Verification items for the finished model (mm, model axes). Round coordinates to 2 decimals unless told otherwise and drop trailing zeros. Write each loop counter-clockwise with the first axis right and the second up, starting at its lowest first coordinate (ties: lowest second). Pieces come first, ordered by that corner, then holes. Notation, with made-up numbers: (48.5, 29) -> (63.5, 29) arc R21 cw to (63.5, 49) -> close; hole circle Ø10 at (3.25, 45). An arc over 180 degrees is marked (long way). Answer as a JSON object with one key per item and string values. Group by question number.
(1) Sectioned sample at A-A on x = 22. Record the cut outline in (y, z), and give its area (3 significant figures).
(2) Sectioned sample at B-B on z = 3.2. Record the cut outline in (x, y), and give its area (3 significant figures).
(3) Sectioned sample at C-C on y = -11.5. Record the cut outline in (x, z).
(4) Scan lines: L1, parallel to Y at x = 17, z = 1.8; L2, parallel to X at y = -11.5, z = 4.5; L3, parallel to X at y = 10.5, z = 2.65. Record each from-to range of solid material in increasing order. Write a range as from..to.
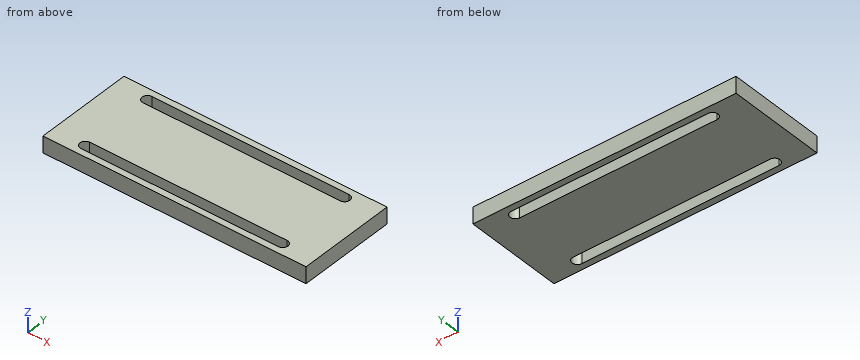
Autodesk Inventor part; units mm, degrees
ref_plane "YZ Plane" through (0, 0, 0) normal (1, 0, 0) x (0, 1, 0)
ref_plane "XZ Plane" through (0, 0, 0) normal (0, 1, 0) x (-1, 0, 0)
ref_plane "XY Plane" through (0, 0, 0) normal (0, 0, 1) x (1, 0, 0)
sketch "スケッチ1" plane through (0, 0, 0) normal (0, 0, 1) x (1, 0, 0)
  line L0 (-40, 15) -> (40, 15)
  line L1 (40, 15) -> (40, -15)
  line L2 (40, -15) -> (-40, -15)
  line L3 (-40, -15) -> (-40, 15)
  point P0 (0, 0)
  dimension "d0" = 80
  dimension "d1" = 40
  dimension "d2" = 30
  dimension "d3" = 15
extrude "押し出し1" add sketch "スケッチ1" along normal blind 5
sketch "スケッチ2" plane through (0, 0, 5) normal (0, 0, 1) x (1, 0, 0)
  line L0 (40, 15) -> (40, -15)
  line L1 (-40, 15) -> (40, 15)
  line L2 (-40, -15) -> (-40, 15)
  line L3 (40, -15) -> (-40, -15)
  line L4 (-30, 13.1) -> (30, 13.1)
  line L5 (30, 13.1) -> (30, 9.9)
  line L6 (30, 9.9) -> (-30, 9.9)
  line L7 (-30, 9.9) -> (-30, 13.1)
  line L8 (-30, -9.9) -> (30, -9.9)
  line L9 (30, -9.9) -> (30, -13.1)
  line L10 (30, -13.1) -> (-30, -13.1)
  line L11 (-30, -13.1) -> (-30, -9.9)
  circle A0 centre (-30, 11.5) radius 1.6
  circle A1 centre (30, 11.5) radius 1.6
  circle A2 centre (-30, -11.5) radius 1.6
  circle A3 centre (30, -11.5) radius 1.6
  point P0 (0, 0)
  dimension "d6" = 5.1
  dimension "d7" = 3.2
  dimension "d8" = 5.1
  dimension "d9" = 3.2
  dimension "d10" = 10
  dimension "d11" = 10
  dimension "d12" = 10
  dimension "d13" = 10
extrude "押し出し2" cut sketch "スケッチ2" against normal through all contours A0 L7 | L4 A1 L6 A0 | L7 A0 | A1 L5 | L5 A1 | A2 L11 | L8 A3 L10 A2 | L11 A2 | A3 L9 | L9 A3
equation "\"d8\" = d6"
equation "\"d9\" = d7"
equation "\"d11\" = d10"
equation "\"d12\" = d10"
equation "\"d13\" = d10"
properties part number "JointA3"
Computed values:
{
 "1": {"outline": "(-15, 0) -> (-13.1, 0) -> (-13.1, 5) -> (-15, 5) -> close; (-9.9, 0) -> (9.9, 0) -> (9.9, 5) -> (-9.9, 5) -> close; (13.1, 0) -> (15, 0) -> (15, 5) -> (13.1, 5) -> close", "area": "118 mm2"},
 "2": {"outline": "(-40, -15) -> (40, -15) -> (40, 15) -> (-40, 15) -> close; hole (-30, -13.1) -> (30, -13.1) arc R1.6 ccw to (30, -9.9) -> (-30, -9.9) arc R1.6 ccw to start; hole (-30, 9.9) -> (30, 9.9) arc R1.6 ccw to (30, 13.1) -> (-30, 13.1) arc R1.6 ccw to start", "area": "2,000 mm2"},
 "3": {"outline": "(-40, 0) -> (-31.6, 0) -> (-31.6, 5) -> (-40, 5) -> close; (31.6, 0) -> (40, 0) -> (40, 5) -> (31.6, 5) -> close"},
 "4": {"L1": "-15..-13.1, -9.9..9.9, 13.1..15", "L2": "-40..-31.6, 31.6..40", "L3": "-40..-31.25, 31.25..40"}
}
